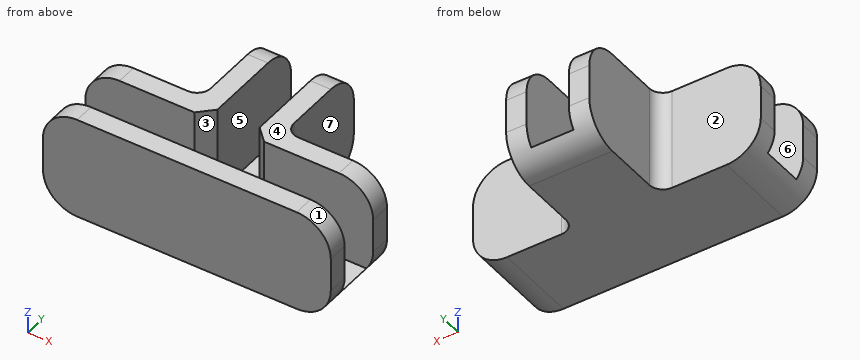
from build123d import *

# Parameters (mm, degrees)
F1_DEPTH     = 2
F2_DEPTH     = 15
F3_R         = 2
F4_T1_DEPTH  = 28
F4_T3_DEPTH  = 28
F4_T5_DEPTH  = 28
F4_T7_DEPTH  = 28
F4_T9_DEPTH  = 37.2
F4_T11_DEPTH = 37.2
F5_R         = 2
F6_SIZE      = 2


# Not quite as in the source:
# - a fillet or chamfer that OpenCascade refuses, or shapes differently, is made with other operations: its cross-section is extruded or revolved along the edge and cut away or added


with BuildPart() as f1:
    # F0 (on Top) → F1 (new body)
    with BuildSketch(Plane.XY):
        Polygon((-21.1, 0), (0, 0), (21.1, 0), (21.1, 6.2), (3.1, 6.2), (3.1, 24.2), (-3.1, 24.2), (-3.1, 6.2), (-21.1, 6.2), align=None)
        Polygon((21.1, 0), (0, 0), (-21.1, 0), (-21.1, -3), (0, -3), (21.1, -3), align=None)
        Polygon((3.1, 6.2), (21.1, 6.2), (21.1, 9.2), (6.1, 9.2), (6.1, 24.2), (3.1, 24.2), align=None)
        Polygon((-21.1, 9.2), (-21.1, 6.2), (-3.1, 6.2), (-3.1, 24.2), (-6.1, 24.2), (-6.1, 9.2), align=None)
    extrude(amount=F1_DEPTH)

    # F0 (on Top) → F2 (join)
    with BuildSketch(Plane.XY):
        Polygon((-21.1, 9.2), (-21.1, 6.2), (-3.1, 6.2), (-3.1, 24.2), (-6.1, 24.2), (-6.1, 9.2), align=None)
        Polygon((3.1, 6.2), (21.1, 6.2), (21.1, 9.2), (6.1, 9.2), (6.1, 24.2), (3.1, 24.2), align=None)
        Polygon((21.1, 0), (0, 0), (-21.1, 0), (-21.1, -3), (0, -3), (21.1, -3), align=None)
    extrude(amount=F2_DEPTH)

    # F3
    f3_edges = [f1.edges().sort_by_distance(p)[0] for p in [
        (6.1, 9.2, 7.5),
    ]]
    fillet(f3_edges, radius=F3_R)

    # F4: fillet of radius 5 on 9 edges, made by hand

    # F4_s2 → F4_t1 (cut)
    with BuildSketch(Plane.XZ.offset(-12.5)):
        with BuildLine():
            ThreePointArc((21.1, 10), (19.6355339059, 13.5355339059), (16.1, 15))
            Line((16.1, 15), (21.1, 15))
            Line((21.1, 15), (21.1, 10))
        make_face()
        with BuildLine():
            ThreePointArc((-21.1, 10), (-19.6355339059, 13.5355339059), (-16.1, 15))
            Line((-16.1, 15), (-21.1, 15))
            Line((-21.1, 15), (-21.1, 10))
        make_face()
    extrude(amount=F4_T1_DEPTH, mode=Mode.SUBTRACT)

    # F4_s4 → F4_t3 (cut)
    with BuildSketch(Plane.XZ.offset(-21.7)):
        with BuildLine():
            ThreePointArc((21.1, 10), (19.6355339059, 13.5355339059), (16.1, 15))
            Line((16.1, 15), (21.1, 15))
            Line((21.1, 15), (21.1, 10))
        make_face()
        with BuildLine():
            ThreePointArc((-21.1, 10), (-19.6355339059, 13.5355339059), (-16.1, 15))
            Line((-16.1, 15), (-21.1, 15))
            Line((-21.1, 15), (-21.1, 10))
        make_face()
    extrude(amount=F4_T3_DEPTH, mode=Mode.SUBTRACT)

    # F4_s6 → F4_t5 (cut)
    with BuildSketch(Plane.YZ.offset(-18.6)):
        with BuildLine():
            ThreePointArc((24.2, 10), (22.7355339059, 13.5355339059), (19.2, 15))
            Line((19.2, 15), (24.2, 15))
            Line((24.2, 15), (24.2, 10))
        make_face()
    extrude(amount=F4_T5_DEPTH, mode=Mode.SUBTRACT)

    # F4_s8 → F4_t7 (cut)
    with BuildSketch(Plane.YZ.offset(-9.4)):
        with BuildLine():
            ThreePointArc((24.2, 10), (22.7355339059, 13.5355339059), (19.2, 15))
            Line((19.2, 15), (24.2, 15))
            Line((24.2, 15), (24.2, 10))
        make_face()
    extrude(amount=F4_T7_DEPTH, mode=Mode.SUBTRACT)

    # F4_s10 → F4_t9 (cut)
    with BuildSketch(Plane.XZ.offset(-21.7)):
        with BuildLine():
            ThreePointArc((-16.1, 0), (-19.6355339059, 1.4644660941), (-21.1, 5))
            Line((-21.1, 5), (-21.1, 0))
            Line((-21.1, 0), (-16.1, 0))
        make_face()
        with BuildLine():
            ThreePointArc((16.1, 0), (19.6355339059, 1.4644660941), (21.1, 5))
            Line((21.1, 5), (21.1, 0))
            Line((21.1, 0), (16.1, 0))
        make_face()
    extrude(amount=F4_T9_DEPTH, mode=Mode.SUBTRACT)

    # F4_s12 → F4_t11 (cut)
    with BuildSketch(Plane.YZ.offset(-18.6)):
        with BuildLine():
            ThreePointArc((19.2, 0), (22.7355339059, 1.4644660941), (24.2, 5))
            Line((24.2, 5), (24.2, 0))
            Line((24.2, 0), (19.2, 0))
        make_face()
    extrude(amount=F4_T11_DEPTH, mode=Mode.SUBTRACT)

    # F5
    f5_edges = [f1.edges().sort_by_distance(p)[0] for p in [
        (-6.1, 9.2, 7.5),
    ]]
    fillet(f5_edges, radius=F5_R)

    # F6
    f6_edges = [f1.edges().sort_by_distance(p)[0] for p in [
        (3.1, 6.2, 8.5),
        (-3.1, 6.2, 8.5),
    ]]
    chamfer(f6_edges, length=F6_SIZE)


solid = f1.part
Verification items for the finished model (mm, model axes). Face numbers are marked on the shaded views. A direction names the side the tool comes from. Give positions to 0.01 mm unless a question says otherwise; leave off trailing zeros. Write each loop counter-clockwise with the first axis right and the second up, starting at its lowest first coordinate (ties: lowest second). Pieces come first, ordered by that corner, then holes. Notation, with made-up numbers: (69, 25) - (111, 25) arc R16 ccw to (111, 43) - close; hole circle Ø11 at (83, -24.5). An arc over 180 degrees is marked (long way). Answer as CSV lines item,"result". Start each with the question number.
1. Sectioned sample at A-A (z = 8.5). Record the boundary of the cut face in (x, y).
2. Draft check along Y on the marked faces 1, 2 and 3. Enter one of: pulls with the +Y half, pulls with the -Y half, needs draft (parallel to the pull), parting line crosses it, or undercut.
3. Sectioned sample at B-B (y = 16). Record the boundary of the cut face in (x, z), then the cut area to 3 significant figures.
4. Set-up check for the marked faces 4, 5, 6 and 7: record each of +Z, -Z, +X, -X, +Y, -Y from which the full face is reachable in a straight line by a thin tool's end or side.
5. Thickness scan on line 1 (Y direction, x = 16, z = 9); line 2 (X direction, y = 22.75, z = 10); line 3 (Z direction, x = 3, y = 2.25). Record the ranges inside material, lowest first.
6. Sectioned sample at D-D (z = 13.25). Record the boundary of the cut face in (x, y).
7. Depth check by flat-ended pin: pin 1 (4 mm diameter, centred on y = 14, z = 7.5, fed in from -X); pin 2 (6.5 mm diameter, centred on y = 17, z = 7.5, fed in from +X); pin 3 (1 mm diameter, centred on x = 8, z = 6.5, fed in from +Y). Enter the tip coordinate at first touch or a pass-through.
8. Sectioned sample at C-C (x = 12). Record the boundary of the cut face in (y, z), then the cut area to 3 significant figures.
Derived:
1,outline,"(-21.1, -3) - (21.1, -3) - (21.1, 0) - (-21.1, 0) - close; (-21.1, 6.2) - (-5.1, 6.2) - (-3.1, 8.2) - (-3.1, 24.2) - (-6.1, 24.2) - (-6.1, 11.2) arc R2 cw to (-8.1, 9.2) - (-21.1, 9.2) - close; (3.1, 8.2) - (5.1, 6.2) - (21.1, 6.2) - (21.1, 9.2) - (8.1, 9.2) arc R2 cw to (6.1, 11.2) - (6.1, 24.2) - (3.1, 24.2) - close"
2,face 1,"needs draft"
2,face 2,"pulls with the +Y half"
2,face 3,"undercut"
3,outline,"(-6.1, 0) - (6.1, 0) - (6.1, 15) - (3.1, 15) - (3.1, 2) - (-3.1, 2) - (-3.1, 15) - (-6.1, 15) - close"
3,area,"102 mm²"
4,face 4,"+Z, +X, -X, +Y, -Y"
4,face 5,"+Z, +Y"
4,face 6,"+Z, +X, -X"
4,face 7,"+Z, -Z, +X, +Y"
5,line 1,"-3 to 0, 6.2 to 9.2"
5,line 2,"-6.1 to -3.1, 3.1 to 6.1"
5,line 3,"0 to 2"
6,outline,"(-19.9, -3) - (19.9, -3) - (19.9, 0) - (-19.9, 0) - close; (-19.9, 6.2) - (-5.1, 6.2) - (-3.1, 8.2) - (-3.1, 23) - (-6.1, 23) - (-6.1, 11.2) arc R2 cw to (-8.1, 9.2) - (-19.9, 9.2) - close; (3.1, 8.2) - (5.1, 6.2) - (19.9, 6.2) - (19.9, 9.2) - (8.1, 9.2) arc R2 cw to (6.1, 11.2) - (6.1, 23) - (3.1, 23) - close"
7,pin 1,"x = -6.1"
7,pin 2,"x = 6.1"
7,pin 3,"y = 9.29"
8,outline,"(-3, 0) - (9.2, 0) - (9.2, 15) - (6.2, 15) - (6.2, 2) - (0, 2) - (0, 15) - (-3, 15) - close"
8,area,"102 mm²"
